Autodesk Inventor part; units mm, degrees
ref_plane "Arbeitsebene3" through (-10.9602, 0, 10.9602) normal (-0.7071, 0, 0.7071) x (0, -1, 0)
ref_plane "XZ Plane" through (0, 0, 0) normal (0, 1, 0) x (-1, 0, 0)
ref_plane "Arbeitsebene2" through (0, 0, 0) normal (-0.7071, 0, 0.7071) x (0, -1, 0)
sketch "Skizze1" plane through (0, 0, 0) normal (0, 1, 0) x (-1, 0, 0)
  circle A0 centre (0, 0) radius 3.14
  circle A1 centre (0, 0) radius 12.7
  circle A2 centre (0, 0) radius 15.5
  circle A3 centre (0, 12.7) radius 1.5
  circle A4 centre (12.7, 0) radius 1.5
  circle A5 centre (0, -12.7) radius 1.5
  circle A6 centre (-12.7, 0) radius 1.5
  dimension "d0" = 6.28
  dimension "d1" = 25.4
  dimension "d2" = 31
  dimension "d3" = 3
  dimension "d4" = 3
  dimension "d5" = 3
  dimension "d6" = 3
extrude "Extrusion1" add sketch "Skizze1" along normal blind 8 contours A4 A1 A5 A6 A3 | A2
ref_plane "Arbeitsebene3" through (-10.9602, 0, 10.9602) normal (-0.7071, 0, 0.7071) x (0, -1, 0)
ref_plane "Arbeitsebene2" through (0, 0, 0) normal (-0.7071, 0, 0.7071) x (0, -1, 0)
sketch "Skizze2" plane through (-10.9602, 0, 10.9602) normal (-0.7071, 0, 0.7071) x (0, -1, 0)
  circle A0 centre (-4, 0) radius 1.475
  line L0 (0, 15.5) -> (0, -15.5)
  point P0 (0, 0)
  dimension "d9" = 2.95
  dimension "d10" = 4
extrude "Extrusion2" cut sketch "Skizze2" against normal blind 16
sketch "Skizze3" plane through (0, 0, 0) normal (0, -1, 0) x (1, 0, 0)
  circle A0 centre (0, 0) radius 15.5
  arc A1 (-11.9125, 6.8258) -> (-6.8258, 11.9125) centre (-10.6066, 10.6066) ccw
  line L0 (0, 0) -> (-15.0003, 15.0003) construction
  line L1 (0, 0) -> (0, 6.573) construction
  arc A2 (-14.4271, 5.6666) -> (-5.6666, 14.4271) centre (0, 0) ccw
  arc A3 (-11.9125, 6.8258) -> (-14.4271, 5.6666) centre (-12.5655, 4.9354) ccw
  arc A4 (-5.6666, 14.4271) -> (-6.8258, 11.9125) centre (-4.9354, 12.5655) ccw
  point P0 (-5.6666, 14.4271)
  point P1 (-14.4271, 5.6666)
  dimension "d13" = 8
  dimension "d14" = 45
  dimension "d15" = 2
  dimension "d18" = 15
extrude "Extrusion3" cut sketch "Skizze3" against normal blind 16 contours A4 A1 A3 A0 picked at (-11.6232, 8.691)
pattern_circular "Runde Anordnung1" count 4 over 360 about axis through (0, 0, 0) along (0, 1, 0) of "Extrusion3"
properties part number "lüfter_flansch"
Read the model definition and answer for the solid it produces. Units are mm, in the model's axes. Give positions to 0.01 mm unless a question says otherwise; leave off trailing zeros. Write each loop counter-clockwise with the first axis right and the second up, starting at its lowest first coordinate (ties: lowest second). Pieces come first, ordered by that corner, then holes. Notation, with made-up numbers: (18.25, 57.5) -> (71.25, 57.5) arc R16 cw to (71.25, 68.5) -> close; hole circle Ø11 at (54, 87.25). An arc over 180 degrees is marked (long way). Answer in a Markdown table with one row per item.
1) Section C-C on y = 4.75 is taken. Give the vertices of the cut face in (x, z), plus the area to 3 significant figures.
Results list:
| item | result |
|---|---|
| outline | (-14.43, -5.67) arc R2 ccw to (-11.91, -6.83) arc R4 cw to (-6.83, -11.91) arc R2 ccw to (-5.67, -14.43) arc R15.5 ccw to (5.67, -14.43) arc R2 ccw to (6.83, -11.91) arc R4 cw to (11.91, -6.83) arc R2 ccw to (14.43, -5.67) arc R15.5 ccw to (14.43, 5.67) arc R2 ccw to (11.91, 6.83) arc R4 cw to (6.83, 11.91) arc R2 ccw to (5.67, 14.43) arc R15.5 ccw to (-5.67, 14.43) arc R2 ccw to (-6.83, 11.91) arc R4 cw to (-7.03, 8.82) -> (-1.13, 2.93) arc R3.14 cw (long way) to (-2.93, 1.13) -> (-8.82, 7.03) arc R4 cw to (-11.91, 6.83) arc R2 ccw to (-14.43, 5.67) arc R15.5 ccw to start; hole circle Ø3 at (-12.7, 0); hole circle Ø3 at (0, -12.7); hole circle Ø3 at (0, 12.7); hole circle Ø3 at (12.7, 0) |
| area | 557 mm^2 |
2) Section A-A on z = 0 is taken. Give the vertices of the cut face in (x, y), plus the area to 3 significant figures.
Results list:
| item | result |
|---|---|
| outline | (-15.5, 0) -> (-14.2, 0) -> (-14.2, 8) -> (-15.5, 8) -> close; (-11.2, 0) -> (-3.14, 0) -> (-3.14, 8) -> (-11.2, 8) -> close; (3.14, 0) -> (11.2, 0) -> (11.2, 8) -> (3.14, 8) -> close; (14.2, 0) -> (15.5, 0) -> (15.5, 8) -> (14.2, 8) -> close |
| area | 150 mm^2 |
3) Section D-D on x = 12.7 is taken. Give the vertices of the cut face in (y, z), plus the area to 3 significant figures.
Results list:
| item | result |
|---|---|
| outline | (0, -6.93) -> (8, -6.93) -> (8, -1.5) -> (0, -1.5) -> close; (0, 1.5) -> (8, 1.5) -> (8, 6.93) -> (0, 6.93) -> close |
| area | 86.9 mm^2 |
4) Each of these flat-tipped pins is pushed along its axis until it touches: pin 1 Ø1 at (y, z) = (3.5, -1) entering from -X; pin 2 Ø1.5 at (y, z) = (4.5, -10.5) entering from +X. Where does it stop, or does it pass through?
Results list:
| item | result |
|---|---|
| pin 1 | x = -15.49 |
| pin 2 | x = 6.7 |
5) Section B-B on x = 0 is taken. Give the vertices of the cut face in (y, z), plus the area to 3 significant figures.
Results list:
| item | result |
|---|---|
| outline | (0, -15.5) -> (8, -15.5) -> (8, -14.2) -> (0, -14.2) -> close; (0, -11.2) -> (8, -11.2) -> (8, -3.14) -> (0, -3.14) -> close; (0, 3.14) -> (8, 3.14) -> (8, 11.2) -> (0, 11.2) -> close; (0, 14.2) -> (8, 14.2) -> (8, 15.5) -> (0, 15.5) -> close |
| area | 150 mm^2 |
6) Straight lines are drawn through the part: line 1 (Z direction, x = 0, y = 2.5); line 2 (X direction, y = 6.5, z = -12.7); line 3 (Z direction, x = -10.5, y = 5). For each, find the intervals that lie inside material, in ascending order. Write a range as [from, to].
Results list:
| item | result |
|---|---|
| line 1 | [-15.5, -14.2], [-11.2, -3.14], [3.14, 11.2], [14.2, 15.5] |
| line 2 | [-6.93, -1.5], [1.5, 6.93] |
| line 3 | [-6.61, 6.61] |
7) Determine the mould class of faces 1 (the cylindrical face through (-9.529, 3.944, 6.755)), 2 (the flat face through (0, 8, 4)), 3 (the cylindrical face through (6.743, 3.944, -13.422)), 4 (the cylindrical face through (-15.5, 3.9, 0.1)) for opening direction X: released by +X, released by -X, zero draft, split by the parting line, or undercut.
Results list:
| item | result |
|---|---|
| face 1 | undercut |
| face 2 | zero draft |
| face 3 | released by +X |
| face 4 | released by -X |
